The listing builds one solid part. Answer for the finished solid, in the listing's coordinates (mm). A direction names the side the tool comes from. Round coordinates to 2 decimals unless told otherwise and drop trailing zeros. Order: outer loops, then holes, each group sorted by start corner. A loop starts at its lowest first (then second) coordinate and runs counter-clockwise, first axis right, second up. Notation, with made-up numbers: (25.5, 60) - (43.5, 60) arc R32 ccw to (43.5, 89) - close; hole circle Ø4 at (-22, -17.75). An arc over 180 degrees is marked (long way). One line per item, written item: value. Start each with the question number.
1. For a pull along Y with two mould halves and no side action, classify faces 4 (the cylindrical face through (-10.316, 108.827, -7.91)), 5 (the flat face through (2, 5.594, -2)), 6 (the flat face through (0, -0.406, 0)) as released by +Y, released by -Y, zero draft, split by the parting line, or undercut.
2. Straight lines are drawn through the part: line 1 (Y direction, x = -5.5, z = -2.25); line 2 (Y direction, x = 7.25, z = -6.5); line 3 (Z direction, x = -4, y = 62.5). For each, find the intervals that lie inside material, in ascending order.
3. Flat-ended cylindrical pins translate along their axes: P1, Ø4, axis at y = 34.5, z = -9.5, coming from the +X side; P2, Ø2, axis at x = -6, y = 58.5, coming from the +Z side; P3, Ø7, axis at y = 74, z = 4, coming from the -X side. Find the tip coordinate at first contact, or state that the pin passes through.
4. A tool of negligible diameter and unlimited length cuts with its end or side. For faces 1 (the flat face through (2, 2.594, 6)), 2 (the cylindrical face through (0, 56, 9)), 3 (the flat face through (-1, 56, -5)), from which of +Z, -Z, +X, -X, +Y, -Y can it reach the whole face along a straight path? Write none if from no direction.
5. Section A-A, the plane y = 33.5 is taken. Give the vertices of the cut face in (x, z), then the cut area to 3 significant figures.
Autodesk Inventor part; units mm, degrees
ref_plane "YZ Plane" through (0, 0, 0) normal (1, 0, 0) x (0, 1, 0)
ref_plane "XZ Plane" through (0, 0, 0) normal (0, 1, 0) x (-1, 0, 0)
ref_plane "XY Plane" through (0, 0, 0) normal (0, 0, 1) x (1, 0, 0)
sketch "Sketch1" plane through (0, 0, 0) normal (0, 0, 1) x (1, 0, 0)
  line L0 (0, 5.5944) -> (0, -0.4056)
  line L1 (0, -0.4056) -> (7.5, -0.4056)
  line L2 (7.5, -0.4056) -> (7.5, 2.5944)
  line L3 (7.5, 2.5944) -> (6, 2.5944)
  line L4 (6, 2.5944) -> (6, 4.5944)
  line L5 (6, 4.5944) -> (10, 4.5944)
  line L6 (10, 4.5944) -> (10, 5.5944)
  line L7 (10, 5.5944) -> (0, 5.5944)
  point P0 (0, 0)
  dimension "d0" = 10
  dimension "d1" = 6
  dimension "d2" = 1
  dimension "d3" = 2
  dimension "d4" = 3
  dimension "d5" = 7.5
revolve "Revolution1" add sketch "Sketch1" angle 360 about axis through (0, 5.5944, 0) along (0, -1, 0)
sketch "Sketch2" plane through (0, 5.5944, 0) normal (0, 1, 0) x (1, 0, 0)
  arc A0 (1, 8) -> (-1, 8) centre (0, 8) ccw
  arc A1 (8, -1) -> (8, 1) centre (8, 0) ccw
  arc A2 (-1, -8) -> (1, -8) centre (0, -8) ccw
  arc A3 (-8, 1) -> (-8, -1) centre (-8, 0) ccw
  line L0 (-1, 8) -> (-1, 1.5)
  line L1 (-1, -1.5) -> (-1, -8)
  line L2 (1, 8) -> (1, 1.5)
  line L3 (1, -1.5) -> (1, -8)
  line L4 (-8, -1) -> (-1.5, -1)
  line L5 (1.5, -1) -> (8, -1)
  line L6 (-8, 1) -> (-1.5, 1)
  line L7 (1.5, 1) -> (8, 1)
  arc A4 (-1.5, 1) -> (-1, 1.5) centre (-1.5, 1.5) ccw
  arc A5 (1, 1.5) -> (1.5, 1) centre (1.5, 1.5) ccw
  arc A6 (-1, -1.5) -> (-1.5, -1) centre (-1.5, -1.5) ccw
  arc A7 (1.5, -1) -> (1, -1.5) centre (1.5, -1.5) ccw
  point P0 (0, 0)
  dimension "d11" = 8
  dimension "d16" = 8
  dimension "d17" = 8
  dimension "d18" = 8
  dimension "d19" = 0.5
extrude "Extrusion1" add sketch "Sketch2" along normal blind 102
sketch "Sketch3" plane through (0, 107.5944, 0) normal (0, 1, 0) x (1, 0, 0)
  circle A0 centre (0, 0) radius 13
  dimension "d22" = 26
extrude "Extrusion2" add sketch "Sketch3" along normal blind 2.5
sketch "Sketch4" plane through (0, 110.0944, 0) normal (0, 1, 0) x (1, 0, 0)
  line L0 (10, -1.5) -> (0, -1.5)
  line L1 (10, 1.5) -> (0, 1.5)
  arc A0 (10, -1.5) -> (10, 1.5) centre (10, 0) ccw
  line L2 (8, 2.7) -> (0, 2.7)
  line L3 (8, 5.7) -> (0, 5.7)
  arc A1 (8, 2.7) -> (8, 5.7) centre (8, 4.2) ccw
  line L4 (0, 6.9) -> (6, 6.9)
  line L5 (0, 9.9) -> (6, 9.9)
  arc A2 (6, 6.9) -> (6, 9.9) centre (6, 8.4) ccw
  line L6 (8, -2.7) -> (0, -2.7)
  line L7 (8, -5.7) -> (0, -5.7)
  arc A3 (8, -5.7) -> (8, -2.7) centre (8, -4.2) ccw
  line L8 (6, -6.9) -> (0, -6.9)
  line L9 (6, -9.9) -> (0, -9.9)
  arc A4 (6, -9.9) -> (6, -6.9) centre (6, -8.4) ccw
  line L10 (-10, -1.5) -> (0, -1.5)
  line L11 (-10, 1.5) -> (0, 1.5)
  arc A5 (-10, 1.5) -> (-10, -1.5) centre (-10, 0) ccw
  line L12 (-8, 2.7) -> (0, 2.7)
  line L13 (-8, 5.7) -> (0, 5.7)
  arc A6 (-8, 5.7) -> (-8, 2.7) centre (-8, 4.2) ccw
  line L14 (0, 6.9) -> (-6, 6.9)
  line L15 (0, 9.9) -> (-6, 9.9)
  arc A7 (-6, 9.9) -> (-6, 6.9) centre (-6, 8.4) ccw
  line L16 (-8, -2.7) -> (0, -2.7)
  line L17 (-8, -5.7) -> (0, -5.7)
  arc A8 (-8, -2.7) -> (-8, -5.7) centre (-8, -4.2) ccw
  line L18 (-6, -6.9) -> (0, -6.9)
  line L19 (-6, -9.9) -> (0, -9.9)
  arc A9 (-6, -6.9) -> (-6, -9.9) centre (-6, -8.4) ccw
  point P0 (0, 0)
  dimension "d25" = 1.5
  dimension "d26" = 1.5
  dimension "d27" = 10
  dimension "d28" = 10
  dimension "d29" = 1.2
  dimension "d30" = 3
  dimension "d31" = 8
  dimension "d32" = 8
  dimension "d33" = 1.2
  dimension "d34" = 6
  dimension "d35" = 6
  dimension "d36" = 3
  dimension "d37" = 1.2
  dimension "d38" = 8
  dimension "d39" = 8
  dimension "d40" = 3
  dimension "d41" = 1.2
  dimension "d42" = 3
  dimension "d43" = 6
  dimension "d44" = 6
extrude "Extrusion3" add sketch "Sketch4" along normal blind 1
fillet "Fillet1" radius 1 20 edges at (7.5, 111.0944, -8.4) (0, 111.0944, -9.9) (-7.5, 111.0944, -8.4) (0, 111.0944, -6.9) (9.5, 111.0944, -4.2) (0, 111.0944, -5.7) (-9.5, 111.0944, -4.2) (0, 111.0944, -2.7) (11.5, 111.0944, 0) (0, 111.0944, -1.5) (-11.5, 111.0944, 0) (0, 111.0944, 1.5) (9.5, 111.0944, 4.2) (0, 111.0944, 2.7) (-9.5, 111.0944, 4.2) (0, 111.0944, 5.7) (7.5, 111.0944, 8.4) (0, 111.0944, 6.9) (-7.5, 111.0944, 8.4) (0, 111.0944, 9.9)
properties part number "Plunger"
Answer list:
1. face 4: zero draft
1. face 5: undercut
1. face 6: released by -Y
2. line 1: y = -0.41 to 5.59, 107.59 to 110.09
2. line 2: y = 4.59 to 5.59, 107.59 to 110.09
2. line 3: z = -1 to 1
3. P1: stops at x = 1
3. P2: stops at z = 1
3. P3: stops at x = -8.87
4. face 1: none
4. face 2: +Z
4. face 3: -Z, -X
5. outline: (-8, -1) - (-1.5, -1) arc R0.5 cw to (-1, -1.5) - (-1, -8) arc R1 ccw to (1, -8) - (1, -1.5) arc R0.5 cw to (1.5, -1) - (8, -1) arc R1 ccw to (8, 1) - (1.5, 1) arc R0.5 cw to (1, 1.5) - (1, 8) arc R1 ccw to (-1, 8) - (-1, 1.5) arc R0.5 cw to (-1.5, 1) - (-8, 1) arc R1 ccw to start
5. area: 66.5 mm²
